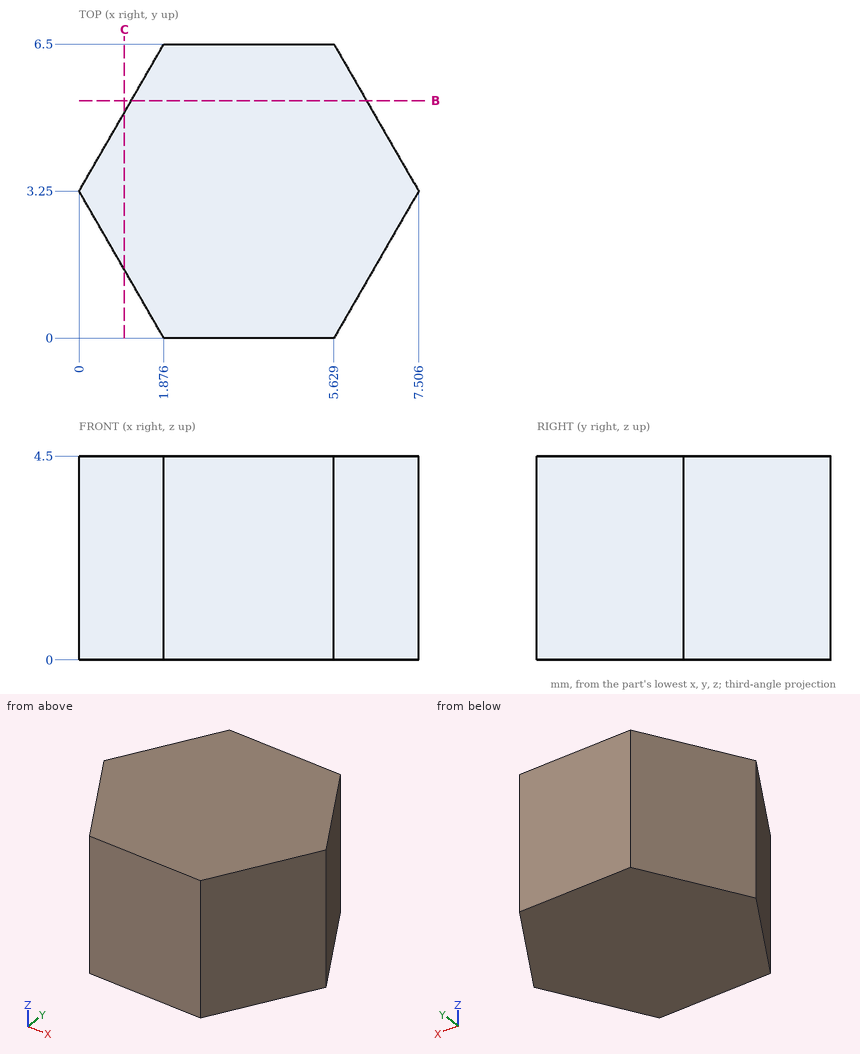
Source: three-view drawing plus pictorial views. Frame: mm from the lowest corner of the part. Give positions to 0.01 mm unless a question says otherwise; leave off trailing zeros. Loops run counter-clockwise (first coordinate to the right, second up) from the corner with the lowest first, then second, coordinate; pieces in that order, holes last. Notation, with made-up numbers: (-19.75, 60) -> (-2.75, 60) arc R20 cw to (-2.75, 81) -> close; hole circle Ø4 at (14, 73). An arc over 180 degrees is marked (long way). Put each result on its own line as item: value. Start each with the question number.
1) Cut plane C-C (x = 1). Return loops of the section in (y, z), then the cut area to 3 significant figures.
2) Cut plane B-B (y = 5.25). Return loops of the section in (x, z) (1 decimal), then the cut area to 3 significant figures.
3) Material intervals for probe 1 along X at (y, z) = (5.5, 2.8) (1 decimal); probe 2 along X at (y, z) = (3, 2.5) (1 decimal); probe 3 along Y at (x, z) = (6.75, 1.95), sorted ascending.
4) Contact query for flat-ended pins moving along their axis: P1, Ø1.5, axis at y = 3, z = 4, coming from the -X side; P2, Ø1, axis at y = 1, z = 2.5, coming from the +X side (1 decimal). Output: stop coordinate, or through.
Results are:
1. outline: (1.52, 0) -> (4.98, 0) -> (4.98, 4.5) -> (1.52, 4.5) -> close
1. area: 15.6 mm2
2. outline: (1.2, 0) -> (6.4, 0) -> (6.4, 4.5) -> (1.2, 4.5) -> close
2. area: 23.4 mm2
3. probe 1: x = 1.3 to 6.2
3. probe 2: x = 0.1 to 7.4
3. probe 3: y = 1.94 to 4.56
4. P1: stops at x = 0
4. P2: stops at x = 6.5
